Geometry: see drawing. Coordinates: mm, zero at the bounding-box minimum. A direction names the side the tool comes from. Give positions to 0.01 mm unless a question says otherwise; leave off trailing zeros. Write each loop counter-clockwise with the first axis right and the second up, starting at its lowest first coordinate (ties: lowest second). Pieces come first, ordered by that corner, then holes. Notation, with made-up numbers: (82.25, 59.25) -> (129.25, 59.25) arc R27 cw to (129.25, 94.25) -> close; hole circle Ø9 at (22, 15). An arc over 180 degrees is marked (long way). Use CSV: the item, a comma, the result in double quotes. Start each with the question number.
1) Section C-C (z = 6). Output: boundary loops of the cut face in (x, y).
2) Section B-B (y = 5). Output: boundary loops of the cut face in (x, z).
3) Contact query for flat-ended pins moving along their axis: P1, Ø3, axis at x = 12.5, y = 5.5, coming from the -Z side; P2, Ø2.5, axis at x = 7.5, y = 5, coming from the -Z side; P3, Ø3.5, axis at x = 7.5, y = 5, coming from the -Z side; P4, Ø1, axis at x = 1.5, z = 4.5, coming from the +Y side. Output: stop coordinate, or through.
4) Set-up query: the marked faces 1, 2, 3 and 4. Return all of +Z, -Z, +X, -X, +Y, -Y with unobstructed straight access to the full face (end or side cutting, diameter ignored); none if empty.
5) Material intervals for line 1 (X direction, y = 31, z = 8.85); line 2 (X direction, y = 31, z = 12.25); line 3 (Y direction, x = 3.15, z = 4), sorted ascending. Write a range as [from, to].
6) Section A-A (x = 7.5). Output: boundary loops of the cut face in (y, z).
7) Draft query along X for the marked faces 5, 6 and 7. Return one class per face: pulls with the +X half, pulls with the -X half, needs draft (parallel to the pull), parting line crosses it, or undercut.
8) Section D-D (x = 3.5). Output: boundary loops of the cut face in (y, z).
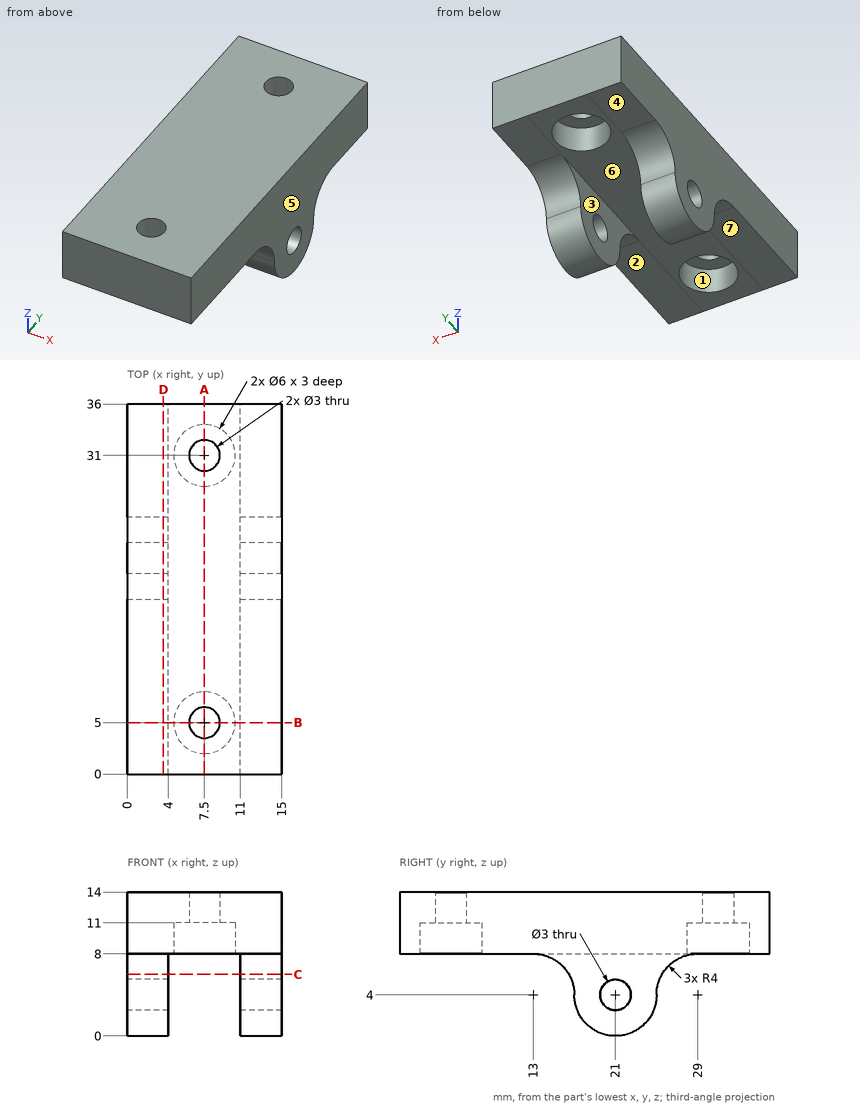
Answers follow:
1,outline,"(0, 16.46) -> (4, 16.46) -> (4, 25.54) -> (0, 25.54) -> close; (11, 16.46) -> (15, 16.46) -> (15, 25.54) -> (11, 25.54) -> close"
2,outline,"(0, 8) -> (4.5, 8) -> (4.5, 11) -> (6, 11) -> (6, 14) -> (0, 14) -> close; (9, 11) -> (10.5, 11) -> (10.5, 8) -> (15, 8) -> (15, 14) -> (9, 14) -> close"
3,P1,"stops at z = 8"
3,P2,"passes through"
3,P3,"stops at z = 11"
3,P4,"stops at y = 25.13"
4,face 1,"-Z"
4,face 2,"-Z, +X, -X, -Y"
4,face 3,"-Z, +Y, -Y"
4,face 4,"-Z, +X, -X, +Y"
5,line 1,"x = [0, 4.5], [10.5, 15]"
5,line 2,"x = [0, 6], [9, 15]"
5,line 3,"y = [17, 19.5], [22.5, 25]"
6,outline,"(0, 8) -> (2, 8) -> (2, 11) -> (3.5, 11) -> (3.5, 14) -> (0, 14) -> close; (6.5, 11) -> (8, 11) -> (8, 8) -> (28, 8) -> (28, 11) -> (29.5, 11) -> (29.5, 14) -> (6.5, 14) -> close; (32.5, 11) -> (34, 11) -> (34, 8) -> (36, 8) -> (36, 14) -> (32.5, 14) -> close"
7,face 5,"pulls with the +X half"
7,face 6,"undercut"
7,face 7,"needs draft"
8,outline,"(0, 8) -> (13, 8) arc R4 cw to (17, 4) arc R4 ccw to (25, 4) arc R4 cw to (29, 8) -> (36, 8) -> (36, 14) -> (0, 14) -> close; hole circle Ø3 at (21, 4)"
